```python
from build123d import *

# Parameters (mm, degrees)
SKETCH1_R           = 7.5
SKETCH1_R_2         = 5
SKETCH1_R_3         = 10
SKETCH1_R_4         = 12.5
SKETCH1_W           = 38.1
SKETCH1_H           = 19.05
BOSS_EXTRUDE2_DEPTH = 6


with BuildPart() as part:
    # Sketch1 → Boss-Extrude2 (new body)
    with BuildSketch(Plane(origin=(0, 0, 0), x_dir=(0, 1, 0), z_dir=(0, 0, 1))):
        Polygon((302.864595387, -433.000855558), (352.864595387, -433.000855558), (352.864595387, -439.000855558), (387.864595387, -439.000855558), (387.864595387, -433.000855558), (437.864595387, -433.000855558), (437.864595387, -439.000855558), (460.664595387, -439.000855558), (460.664595387, -433.000855558), (510.664595387, -433.000855558), (510.664595387, -439.000855558), (545.664595387, -439.000855558), (545.664595387, -433.000855558), (595.664595387, -433.000855558), (595.664595387, -350.737424545), (601.664595387, -350.737424545), (601.664595387, -280.737424545), (595.664595387, -280.737424545), (595.664595387, -179.400855558), (601.664595387, -179.400855558), (601.664595387, -87.636640664), (595.664595387, -87.636640664), (595.664595387, 15.599144442), (601.664595387, 15.599144442), (601.664595387, 85.599144442), (595.664595387, 85.599144442), (595.664595387, 100.599144442), (595.664595387, 170.599144442), (525.664595387, 170.599144442), (372.864595387, 170.599144442), (302.864595387, 170.599144442), (302.864595387, 100.599144442), (302.864595387, 85.599144442), (296.864595387, 85.599144442), (296.864595387, 15.599144442), (302.864595387, 15.599144442), (302.864595387, -89.000855558), (296.864595387, -89.000855558), (296.864595387, -179.400855558), (302.864595387, -179.400855558), (302.864595387, -284.000855558), (296.864595387, -284.000855558), (296.864595387, -354.000855558), (302.864595387, -354.000855558), align=None)
        with Locations(Location((450.664595387, 90.599144442, 0), (0, 0, 270))):
            Circle(SKETCH1_R, mode=Mode.SUBTRACT)
        with Locations(Location((322.864595387, -194.000855558, 0), (0, 0, 270))):
            Circle(SKETCH1_R_2, mode=Mode.SUBTRACT)
        with Locations(Location((508.701533875, -309.936805208, 0), (0, 0, 270))):
            Circle(SKETCH1_R, mode=Mode.SUBTRACT)
        with Locations(Location((368.382345964, -311.573747263, 0), (0, 0, 90))):
            Circle(SKETCH1_R, mode=Mode.SUBTRACT)
        with Locations(Location((377.864595387, -89.400855558, 0), (0, 0, 270))):
            Circle(SKETCH1_R_3, mode=Mode.SUBTRACT)
        with Locations(Location((520.664595387, -159.400855558, 0), (0, 0, 270))):
            Circle(SKETCH1_R_3, mode=Mode.SUBTRACT)
        with Locations(Location((520.664595387, -378.000855558, 0), (0, 0, 270))):
            Circle(SKETCH1_R_4, mode=Mode.SUBTRACT)
        Polygon((480.935500713, -15.863437319), (489.068063381, -21.682494326), (493.141403286, -15.989700458), (485.008840618, -10.170643451), align=None, mode=Mode.SUBTRACT)
        Polygon((525.664595387, -47.868250858), (529.737935292, -42.17545699), (521.605372624, -36.356399983), (517.532032719, -42.04919385), align=None, mode=Mode.SUBTRACT)
        with Locations((361.914595387, -398.475855558)):
            Rectangle(SKETCH1_W, SKETCH1_H, mode=Mode.SUBTRACT)
    extrude(amount=BOSS_EXTRUDE2_DEPTH)


solid = part.part
```
Can you work these out from the model? Positions are in its coordinate system, mm. Coordinates: 2 decimals unless noted, no trailing zeros. Loops run counter-clockwise (first coordinate to the right, second up) from the corner with the lowest first, then second, coordinate; pieces in that order, holes last. Notation, with made-up numbers: M -39.75,4 L -23.75,4 A17 ccw -23.75,37 Z; hole C 82,13.25 d5. An arc over 180 degrees is marked long. Put each result on its own line as item: value. Start each with the question number.
(1) Will these pins go through, and if not, where does the flat tip stop? pin 1 Ø1.8 at (y, z) = (300, 2) entering from -X; pin 2 Ø3 at (x, z) = (-145.5, 2.5) entering from -Y; pin 3 Ø3 at (x, z) = (26.5, 3.5) entering from +Y.
(2) Imagine slicing it at C-C on x = -117. List the corners of the cut face in (y, z) for me, and give its area (3 significant figures).
(3) We'd pull the mould along Y, two halves only. Please class faces 1 (the face through (130, 447, 0)), 2 (the face through (313.4, 502.05, 2.96)): +Y half, -Y half, draft (parallel to the pull), parting line (faces both ways), or undercut.
(4) Imagine slicing it at A-A on x = 158. List the corners of the cut face in (y, z) for me.
(5) I need wall thicknesses on probe 1 along X at (y, z) = (379, 4.3); probe 2 along Y at (x, z) = (-11, 4.85); probe 3 along X at (y, z) = (579, 4.15). Which ranges of each line are inside material? Lowest first, please.
(6) Imagine slicing it at B-B on z = 1.9. Give the number of separate pieces and of enclosed holes in the cut face, and give its area (3 significant figures).
Worked answers:
1. pin 1: stops at x = -85.6
1. pin 2: stops at y = 302.86
1. pin 3: stops at y = 595.66
2. outline: M 302.86,0 L 595.66,0 L 595.66,6 L 302.86,6 Z
2. area: 1,760 mm2
3. face 1: draft
3. face 2: undercut
4. outline: M 296.86,0 L 510.76,0 L 510.76,6 L 296.86,6 Z; M 530.57,0 L 601.66,0 L 601.66,6 L 530.57,6 Z
5. probe 1: x = -170.6 to 79.47, 99.34 to 388.95, 408 to 439
5. probe 2: y = 302.86 to 595.66
5. probe 3: x = -170.6 to 433
6. separate pieces: 1
6. enclosed holes: 10
6. area: 177,000 mm2
